```python
from build123d import *

# Parameters (mm, degrees)
BOSS_EXTRUDE1_DEPTH = 3.175
FILLET1_R           = 6.35
SKETCH3_R           = 3.302
CUT_EXTRUDE1_DEPTH  = 3.175
SKETCH4_W           = 3.175
SKETCH4_H           = 4.60375
CUT_EXTRUDE2_DEPTH  = 3.175


with BuildPart() as part:
    # Sketch1 → Boss-Extrude1 (new body)
    with BuildSketch(Plane.XY):
        Polygon((0, -9.525), (6.35, -9.525), (31.75, -22.225), (31.75, 9.525), (0, 9.525), align=None)
    extrude(amount=BOSS_EXTRUDE1_DEPTH)

    # Fillet1
    fillet1_edges = [part.edges().sort_by_distance(p)[0] for p in [
        (31.75, 9.525, 1.5875),
        (31.75, -22.225, 1.5875),
        (6.35, -9.525, 1.5875),
    ]]
    fillet(fillet1_edges, radius=FILLET1_R)

    # Sketch3 → Cut-Extrude1 (cut)
    with BuildSketch(Plane.XY.offset(3.175)):
        with Locations((21.588299978, -10.315871599)):
            Circle(SKETCH3_R)
    extrude(amount=-CUT_EXTRUDE1_DEPTH, mode=Mode.SUBTRACT)

    # Sketch4 → Cut-Extrude2 (cut)
    with BuildSketch(Plane.XY.offset(3.175)):
        with Locations((1.5875, 7.223125)):
            Rectangle(SKETCH4_W, SKETCH4_H)
        with Locations((1.5875, -7.223125)):
            Rectangle(SKETCH4_W, SKETCH4_H)
    extrude(amount=-CUT_EXTRUDE2_DEPTH, mode=Mode.SUBTRACT)


solid = part.part
```
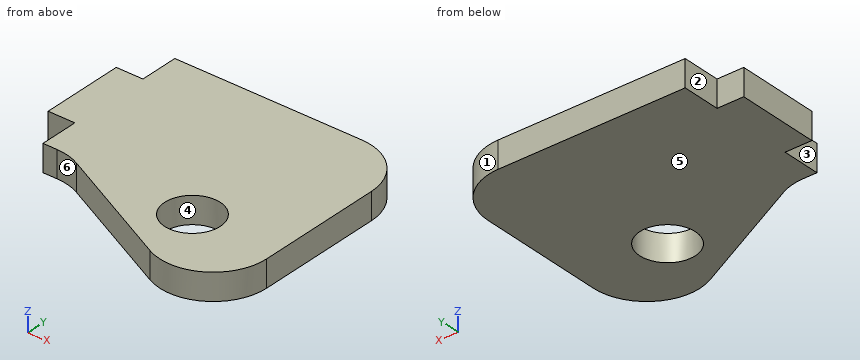
The model under review builds one solid part; all positions refer to its coordinate system, in mm. Face numbers are marked on the shaded views. A direction names the side the tool comes from. Round coordinates to 2 decimals unless told otherwise and drop trailing zeros. Write each loop counter-clockwise with the first axis right and the second up, starting at its lowest first coordinate (ties: lowest second). Pieces come first, ordered by that corner, then holes. Notation, with made-up numbers: (21.25, 69) - (36.25, 69) arc R20 cw to (36.25, 75) - close; hole circle Ø6 at (51.5, -24.5). An arc over 180 degrees is marked (long way). One line per question, with ' | ' between items.
Item 1: The part is to be moulded in two halves that separate along Y. For the marked faces 4, 5 and 6, say which applies: pulls with the +Y half, pulls with the -Y half, needs draft (parallel to the pull), parting line crosses it, or undercut.
Resolved:
face 4: undercut | face 5: needs draft | face 6: pulls with the -Y half
Item 2: For P1, Ø0.5, axis at x = 3.5, z = 1.5, coming from the -Y side (3 decimals); P2, Ø1.6, axis at x = 2, z = 1, coming from the +Y side; P3, Ø1, axis at x = 1.5, z = 2, coming from the -Y side; P4, Ø10.5, axis at x = 21.59, y = -10.32, coming from the -Z side, all flat-tipped, find the tip position at first contact; note any pin that passes through.
Resolved:
P1: stops at y = -9.525 | P2: stops at y = 4.92 | P3: stops at y = -4.92 | P4: stops at z = 0
Item 3: Add section C-C, the plane z = 0.4. Give the boundary of the cut face in (x, y) (3 decimals), then the cut area to 3 significant figures.
Resolved:
outline: (0, -4.921) - (3.175, -4.921) - (3.175, -9.525) - (4.851, -9.525) arc R6.35 cw to (7.691, -10.195) - (22.56, -17.63) arc R6.35 ccw to (31.75, -11.95) - (31.75, 3.175) arc R6.35 ccw to (25.4, 9.525) - (3.175, 9.525) - (3.175, 4.921) - (0, 4.921) - close; hole circle Ø6.604 at (21.588, -10.316) | area: 670 mm2
Item 4: Add section A-A, the plane y = -13. Give the boundary of the cut face in (x, z) (3 decimals), then the cut area to 3 significant figures.
Resolved:
outline: (13.3, 0) - (19.665, 0) - (19.665, 3.175) - (13.3, 3.175) - close; (23.511, 0) - (31.663, 0) - (31.663, 3.175) - (23.511, 3.175) - close | area: 46.1 mm2
Item 5: For the marked faces 1, 2 and 3, list the 3-axis set-ups (+Z, -Z, +X, -X, +Y, -Y) from which the entire face can be reached by the end or side of a thin tool; tool diameter is ignored.
Resolved:
face 1: +Z, -Z, +X, +Y | face 2: +Z, -Z, -X, +Y | face 3: +Z, -Z, -X, -Y
Item 6: To check wall thickness, follow probe 1 along Y at (x, z) = (3.5, 1.1) (3 decimals); probe 2 along Y at (x, z) = (21, 1.75) (3 decimals); probe 3 along X at (y, z) = (-5.5, 2.2) (3 decimals). State the ranges of each line that lie inside material, in increasing order.
Resolved:
probe 1: y = -9.525 to 9.525 | probe 2: y = -16.85 to -13.565, -7.067 to 9.525 | probe 3: x = 3.175 to 31.75
Item 7: Add section D-D, the plane x = 4.5. Give the boundary of the cut face in (y, z) (3 decimals), then the cut area to 3 significant figures.
Resolved:
outline: (-9.525, 0) - (9.525, 0) - (9.525, 3.175) - (-9.525, 3.175) - close | area: 60.5 mm2
Item 8: Add section B-B, the plane x = 19. Give the boundary of the cut face in (y, z) (3 decimals), then the cut area to 3 significant figures.
Resolved:
outline: (-15.85, 0) - (-12.366, 0) - (-12.366, 3.175) - (-15.85, 3.175) - close; (-8.266, 0) - (9.525, 0) - (9.525, 3.175) - (-8.266, 3.175) - close | area: 67.5 mm2
